Verification items for the finished model (mm, model axes). Give positions to 0.01 mm unless a question says otherwise; leave off trailing zeros. Order: outer loops, then holes, each group sorted by start corner. A loop starts at its lowest first (then second) coordinate and runs counter-clockwise, first axis right, second up.
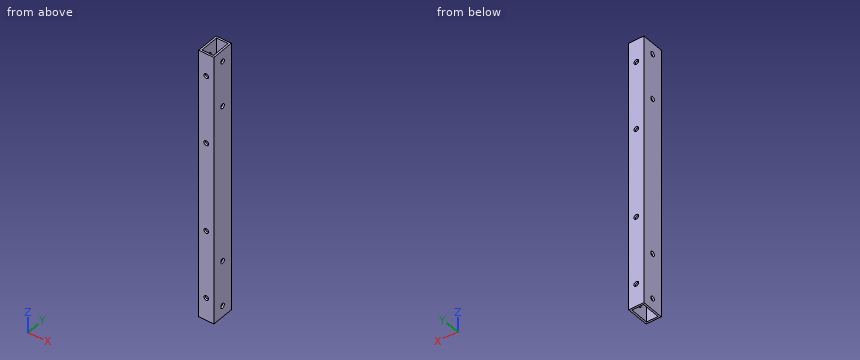
Autodesk Inventor part; units mm, degrees
ref_plane "YZ Plane" through (0, 0, 0) normal (1, 0, 0) x (0, 1, 0)
ref_plane "XZ Plane" through (0, 0, 0) normal (0, 1, 0) x (-1, 0, 0)
ref_plane "XY Plane" through (0, 0, 0) normal (0, 0, 1) x (1, 0, 0)
sketch "スケッチ1" plane through (0, 0, 0) normal (0, 1, 0) x (-1, 0, 0)
  line L0 (0, 0) -> (10, 0)
  line L1 (10, 0) -> (10, 178.952)
  line L2 (10, 178.952) -> (0, 178.952)
  line L3 (0, 178.952) -> (0, 0)
  dimension "d0" = 10
  dimension "d1" = 178.952
extrude "押し出し1" add sketch "スケッチ1" along normal blind 15
shell "シェル1" thickness 1.2 removed faces 2 at (-3.3333, 5, 0) at (-6.6667, 5, 178.952)
sketch "スケッチ2" plane through (-10, 0, 0) normal (-1, 0, 0) x (0, 0, 1)
  line L0 (0, 1.2) -> (0, 13.8)
  line L1 (0, 7.5) -> (178.952, 7.5)
  line L2 (178.952, 1.2) -> (178.952, 13.8)
  point P0 (0, 0)
  point P1 (171.452, 7.5)
  point P2 (141.452, 7.5)
  point P3 (7.5, 7.5)
  point P4 (37.5, 7.5)
  dimension "d5" = 7.5
  dimension "d6" = 30
  dimension "d7" = 7.5
  dimension "d8" = 30
hole "穴1" at (-10, 7.5, 171.452) at (-10, 7.5, 141.452) at (-10, 7.5, 7.5) at (-10, 7.5, 37.5) direction (1, 0, 0) diameter 3.1 end through all
sketch "スケッチ3" plane through (0, 15, 0) normal (0, 1, 0) x (1, 0, 0)
  line L0 (0, 0) -> (-10, 0)
  line L1 (-5, 0) -> (-5, -178.952)
  line L2 (-10, -178.952) -> (0, -178.952)
  point P0 (-5, -15)
  point P1 (-5, -60)
  point P2 (-5, -163.952)
  point P3 (-5, -118.952)
  dimension "d16" = 15
  dimension "d17" = 45
  dimension "d18" = 15
  dimension "d19" = 45
hole "穴2" at (-5, 15, 15) at (-5, 15, 60) at (-5, 15, 163.952) at (-5, 15, 118.952) direction (0, -1, 0) diameter 3.1 end through all
sketch "スケッチ4" plane through (0, 15, 0) normal (0, 1, 0) x (1, 0, 0)
  circle A0 centre (-5, -118.952) radius 1.55
  circle A1 centre (-5, -60) radius 1.55
  line L0 (-5, -118.952) -> (-5, -60)
  line L1 (-5, -89.476) -> (-135, -89.476)
  circle A2 centre (-70, -90.476) radius 88
  line L2 (-70, -90.476) -> (-7.7746, -28.2506)
  line L3 (-5, -90.476) -> (-135, -90.476)
  point P0 (0, 0)
  point P1 (-132.2254, -28.2506)
  point P2 (-132.2254, -152.7014)
  point P3 (-7.7746, -152.7014)
  dimension "d30" = 176
  dimension "d27" = 130
  dimension "d34" = 360
  dimension "d47" = 1
hole "穴3" [suppressed]
properties part number "base_pipe1" material "アルミニウム 6061"
(1) Section check C-C, the plane z = 31. Enter the section's corners in (x, y).
Solved:
outline: (-10, 0) - (0, 0) - (0, 15) - (-10, 15) - close; hole (-8.8, 1.2) - (-1.2, 1.2) - (-1.2, 13.8) - (-8.8, 13.8) - close
(2) Scan lines: line 1 (Z direction, x = -5, y = 0.45); line 2 (Z direction, x = -9.5, y = 7.5); line 3 (X direction, y = 4.5, z = 96). Record each from-to range of solid material in increasing order.
Solved:
line 1: z = 0 to 13.45, 16.55 to 58.45, 61.55 to 117.4, 120.5 to 162.4, 165.5 to 178.95
line 2: z = 0 to 5.95, 9.05 to 35.95, 39.05 to 139.9, 143 to 169.9, 173 to 178.95
line 3: x = -10 to -8.8, -1.2 to 0
(3) Section check A-A, the plane y = 2.75. Enter the section's corners in (x, z), then the cut area to 3 significant figures.
Solved:
outline: (-10, 0) - (-8.8, 0) - (-8.8, 178.95) - (-10, 178.95) - close; (-1.2, 0) - (0, 0) - (0, 178.95) - (-1.2, 178.95) - close
area: 429 mm2
(4) Section check B-B, the plane z = 7.5. Enter the section's corners in (x, y), then the cut area to 3 significant figures.
Solved:
outline: (-10, 0) - (0, 0) - (0, 5.95) - (-1.2, 5.95) - (-1.2, 1.2) - (-8.8, 1.2) - (-8.8, 5.95) - (-10, 5.95) - close; (-10, 9.05) - (-8.8, 9.05) - (-8.8, 13.8) - (-1.2, 13.8) - (-1.2, 9.05) - (0, 9.05) - (0, 15) - (-10, 15) - close
area: 46.8 mm2
